Read the model definition and answer for the solid it produces. Units are mm, in the model's axes. Coordinates: 2 decimals unless noted, no trailing zeros. Order: outer loops, then holes, each group sorted by start corner. A loop starts at its lowest first (then second) coordinate and runs counter-clockwise, first axis right, second up. Notation, with made-up numbers: M 16,47 L 68,47 A27 ccw 68,81 Z; hole C 51.5,80 d11. An arc over 180 degrees is marked long. Use a Markdown table: item, result. Add a question column.
1) Find section D-D on y = -4.5. Write down the section's boundary in (x, z).
2) Each of these flat-tipped pins is pushed along its axis until it touches: pin 1 Ø3 at (x, z) = (9, 2) entering from -Y; pin 2 Ø2 at (x, z) = (2.5, 1) entering from +Y; pin 3 Ø3 at (x, z) = (-6.5, 4) entering from -Y. Where does it stop, or does it pass through?
3) The mould has two halves that part along X. Classify faces 1 (the face through (-12.5, 0, 2)), 2 (the face through (-0.275, -37.497, 2.479)), 3 (the face through (-8.16, 32.49, 2.54)): released by +X, released by -X, zero draft, split by the parting line, or undercut.
4) Find section C-C on y = 21.5. Write down the section's boundary in (x, z), plus the area to 3 significant figures.
5) Find the intervals of material crossed by probe 1 along Y at (x, z) = (0, 2.2) (3 decimals); probe 2 along Y at (x, z) = (0, 0.25) (3 decimals); probe 3 along X at (y, z) = (24.5, 3.7), in increasing order. Write a range as [from, to].
6) Find section A-A on x = 0. Write down the section's boundary in (y, z) (3 decimals), plus the area to 3 significant figures.
7) Find section B-B on z = 2. Write down the section's boundary in (x, y) (3 decimals).
from build123d import *

# Parameters (mm, degrees)
F1_DEPTH = 5
F2_R     = 11.075
F3_DEPTH = 25
F4_R     = 1


with BuildPart() as f1:
    # F0 (on Top) → F1 (new body)
    with BuildSketch(Plane.XY):
        with BuildLine():
            ThreePointArc((-12.5, -25), (0, -37.5), (12.5, -25))
            Line((12.5, -25), (-12.5, -25))
        make_face()
        with BuildLine():
            Line((-12.5, 25), (12.5, 25))
            ThreePointArc((12.5, 25), (0, 37.5), (-12.5, 25))
        make_face()
        with BuildLine():
            Line((12.5, -25), (12.5, 0))
            ThreePointArc((12.5, 0), (8.838835, -8.838835), (0, -12.5))
            ThreePointArc((0, -12.5), (8.838835, -16.161165), (12.5, -25))
        make_face()
        with BuildLine():
            ThreePointArc((-12.5, -25), (-8.838835, -16.161165), (0, -12.5))
            ThreePointArc((0, -12.5), (-8.838835, -8.838835), (-12.5, 0))
            Line((-12.5, 0), (-12.5, -25))
        make_face()
        with BuildLine():
            ThreePointArc((-12.5, 0), (-8.838835, 8.838835), (0, 12.5))
            ThreePointArc((0, 12.5), (-8.838835, 16.161165), (-12.5, 25))
            Line((-12.5, 25), (-12.5, 0))
        make_face()
        with BuildLine():
            ThreePointArc((0, 12.5), (8.838835, 8.838835), (12.5, 0))
            Line((12.5, 0), (12.5, 25))
            ThreePointArc((12.5, 25), (8.838835, 16.161165), (0, 12.5))
        make_face()
        with BuildLine():
            ThreePointArc((-12.5, 25), (-8.838835, 16.161165), (0, 12.5))
            ThreePointArc((0, 12.5), (8.838835, 16.161165), (12.5, 25))
            Line((12.5, 25), (-12.5, 25))
        make_face()
        with BuildLine():
            ThreePointArc((12.5, -25), (8.838835, -16.161165), (0, -12.5))
            ThreePointArc((0, -12.5), (-8.838835, -16.161165), (-12.5, -25))
            Line((-12.5, -25), (12.5, -25))
        make_face()
        with BuildLine():
            ThreePointArc((0, -12.5), (8.838835, -8.838835), (12.5, 0))
            ThreePointArc((12.5, 0), (8.838835, 8.838835), (0, 12.5))
            ThreePointArc((0, 12.5), (-8.838835, 8.838835), (-12.5, 0))
            ThreePointArc((-12.5, 0), (-8.838835, -8.838835), (0, -12.5))
        make_face()
    extrude(amount=F1_DEPTH)

    # F2 (on face) → F3 (cut)
    with BuildSketch(Plane.XY.offset(5)):
        with Locations((0, 25)):
            Circle(F2_R)
        Circle(F2_R)
        with Locations((0, -25)):
            Circle(F2_R)
    extrude(amount=-F3_DEPTH, mode=Mode.SUBTRACT)

    # F4
    f4_edges = [f1.edges().sort_by_distance(p)[0] for p in [
        (12.5, 0, 5),
        (0, 37.5, 5),
        (-12.5, 0, 5),
        (-12.5, -25, 2.5),
        (-12.5, 0, 0),
        (-12.5, 25, 2.5),
        (12.5, 0, 0),
    ]]
    fillet(f4_edges, radius=F4_R)


solid = f1.part
Check result:
| question | item | result |
|---|---|---|
| 1 | outline | M -12.5,1 A1 ccw -11.5,0 L -10.12,0 L -10.12,5 L -11.5,5 A1 ccw -12.5,4 Z; M 10.12,0 L 11.5,0 A1 ccw 12.5,1 L 12.5,4 A1 ccw 11.5,5 L 10.12,5 Z |
| 2 | pin 1 | stops at y = -35 |
| 2 | pin 2 | stops at y = 37.41 |
| 2 | pin 3 | stops at y = -36.46 |
| 3 | face 1 | released by -X |
| 3 | face 2 | split by the parting line |
| 3 | face 3 | undercut |
| 4 | outline | M -12.5,1 A1 ccw -11.5,0 L -10.51,0 L -10.51,5 L -11.5,5 A1 ccw -12.5,4 Z; M 10.51,0 L 11.5,0 A1 ccw 12.5,1 L 12.5,4 A1 ccw 11.5,5 L 10.51,5 Z |
| 4 | area | 19.1 mm2 |
| 5 | probe 1 | y = [-37.5, -36.075], [-13.925, -11.075], [11.075, 13.925], [36.075, 37.5] |
| 5 | probe 2 | y = [-37.161, -36.075], [-13.925, -11.075], [11.075, 13.925], [36.075, 37.161] |
| 5 | probe 3 | x = [-12.5, -11.06], [11.06, 12.5] |
| 6 | outline | M -37.5,1 A1 ccw -36.5,0 L -36.075,0 L -36.075,5 L -36.5,5 A1 ccw -37.5,4 Z; M -13.925,0 L -11.075,0 L -11.075,5 L -13.925,5 Z; M 11.075,0 L 13.925,0 L 13.925,5 L 11.075,5 Z; M 36.075,0 L 36.5,0 A1 ccw 37.5,1 L 37.5,4 A1 ccw 36.5,5 L 36.075,5 Z |
| 6 | area | 41.9 mm2 |
| 7 | outline | M -12.5,-25 A12.5 ccw 12.5,-25 L 12.5,25 A12.5 ccw -12.5,25 Z; hole C 0,-25 d22.15; hole C 0,0 d22.15; hole C 0,25 d22.15 |
